Geometry check sheet. Reference: the model listing, model coordinates, mm. Face numbers are marked on the shaded views. A direction names the side the tool comes from. Coordinates: 2 decimals unless noted, no trailing zeros. Write each loop counter-clockwise with the first axis right and the second up, starting at its lowest first coordinate (ties: lowest second). Pieces come first, ordered by that corner, then holes. Notation, with made-up numbers: (0.5, 52) -> (5.5, 52) arc R28 cw to (5.5, 82) -> close; hole circle Ø9 at (-29, -38). An arc over 180 degrees is marked (long way). Answer as CSV lines item,"result".
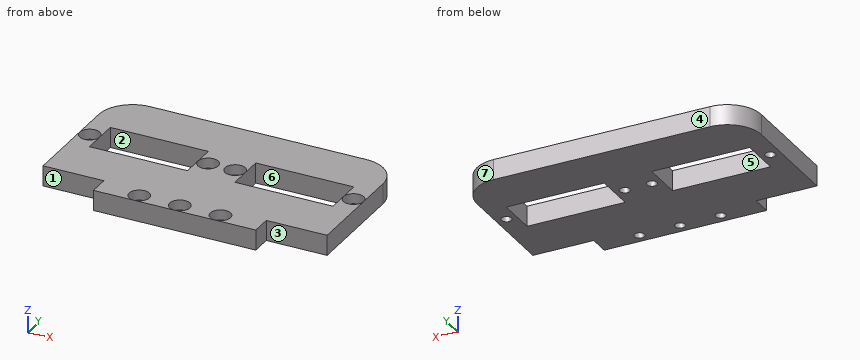
```python
from build123d import *

# Parameters (mm, degrees)
ESQUISSE2_W             = 84
ESQUISSE2_H             = 48
BOSS_EXTRU_1_DEPTH      = 6
ESQUISSE3_R             = 1.5
ESQUISSE3_W             = 18
ESQUISSE3_H             = 6
ESQUISSE3_W_2           = 29
ESQUISSE3_H_2           = 12
ENL_V_MAT_EXTRU_1_DEPTH = 6
ESQUISSE4_R             = 2.995
ENL_V_MAT_EXTRU_2_DEPTH = 3
CONG_1_R                = 10


with BuildPart() as part:
    # Esquisse2 → Boss.-Extru.1 (new body)
    with BuildSketch(Plane.XY):
        with Locations((10.587382635, 10.131926121)):
            Rectangle(ESQUISSE2_W, ESQUISSE2_H)
    extrude(amount=BOSS_EXTRU_1_DEPTH)

    # Esquisse3 → Enlèv. mat.-Extru.1 (cut)
    with BuildSketch(Plane.XY.offset(6)):
        with Locations((-28.412617365, 13.131926121)):
            Circle(ESQUISSE3_R)
        with Locations((49.587382635, 13.131926121)):
            Circle(ESQUISSE3_R)
        with Locations((6.587382635, 13.131926121)):
            Circle(ESQUISSE3_R)
        with Locations((14.587382635, 13.131926121)):
            Circle(ESQUISSE3_R)
        with Locations((-1.412617365, -10.868073879)):
            Circle(ESQUISSE3_R)
        with Locations(Location((22.587382635, -10.868073879, 0), (0, 0, 180))):
            Circle(ESQUISSE3_R)
        with Locations((10.587382635, -10.868073879)):
            Circle(ESQUISSE3_R)
        with Locations((-22.412617365, -10.868073879)):
            Rectangle(ESQUISSE3_W, ESQUISSE3_H)
        with Locations((43.587382635, -10.868073879)):
            Rectangle(ESQUISSE3_W, ESQUISSE3_H)
        with Locations((-10.912617365, 13.131926121)):
            Rectangle(ESQUISSE3_W_2, ESQUISSE3_H_2)
        with Locations((32.087382635, 13.131926121)):
            Rectangle(ESQUISSE3_W_2, ESQUISSE3_H_2)
    extrude(amount=-ENL_V_MAT_EXTRU_1_DEPTH, mode=Mode.SUBTRACT)

    # Esquisse4 → Enlèv. mat.-Extru.2 (cut)
    with BuildSketch(Plane.XY.offset(6)):
        with Locations((-1.412617365, -10.868073879)):
            Circle(ESQUISSE4_R)
        with Locations((22.587382635, -10.868073879)):
            Circle(ESQUISSE4_R)
        with Locations((10.587382635, -10.868073879)):
            Circle(ESQUISSE4_R)
        with Locations((-28.412617365, 13.131926121)):
            Circle(ESQUISSE4_R)
        with Locations((6.587382635, 13.131926121)):
            Circle(ESQUISSE4_R)
        with Locations((14.587382635, 13.131926121)):
            Circle(ESQUISSE4_R)
        with Locations((49.587382635, 13.131926121)):
            Circle(ESQUISSE4_R)
    extrude(amount=-ENL_V_MAT_EXTRU_2_DEPTH, mode=Mode.SUBTRACT)

    # Congé1
    cong_1_edges = [part.edges().sort_by_distance(p)[0] for p in [
        (-31.412617365, 34.131926121, 3),
        (52.587382635, 34.131926121, 3),
    ]]
    fillet(cong_1_edges, radius=CONG_1_R)


solid = part.part
```
Item 1: Cross-section at C-C, the plane y = 31. Record the cut outline in (x, z), plus the area to 3 significant figures.
Responses:
outline,"(-28.68, 0) -> (49.86, 0) -> (49.86, 6) -> (-28.68, 6) -> close"
area,"471 mm2"
Item 2: Depth check by flat-ended pin: pin 1 Ø5 at (x, y) = (-1, -11) entering from +Z; pin 2 Ø1.5 at (x, z) = (-23, 1) entering from +Y. Enter the tip coordinate at first touch or a pass-through.
Responses:
pin 1,"stops at z = 3"
pin 2,"stops at y = 34.1"
Item 3: Thickness scan on probe 1 along Y at (x, z) = (3.5, 4.35); probe 2 along Y at (x, z) = (-18.5, 2.4); probe 3 along X at (y, z) = (10, 0.85). Record the ranges inside material, lowest first.
Responses:
probe 1,"y = -13.87 to 7.13, 19.13 to 34.13"
probe 2,"y = -7.87 to 7.13, 19.13 to 34.13"
probe 3,"x = -31.41 to -25.41, 3.59 to 17.59, 46.59 to 52.59"
Item 4: Set-up check for the marked faces 1, 2 and 3: record each of +Z, -Z, +X, -X, +Y, -Y from which the full face is reachable in a straight line by a thin tool's end or side.
Responses:
face 1,"+Z, -Z, -X, -Y"
face 2,"+Z, -Z"
face 3,"+Z, -Z, +X, -Y"
Item 5: Cross-section at B-B, the plane z = 2.2. Count the separate pieces of the cut face and the enclosed holes in it, plus the area to 3 significant figures.
Responses:
separate pieces,"1"
enclosed holes,"9"
area,"3,030 mm2"
Item 6: Release check for a two-part mould opening along X. For the marked faces 4, 5, 6 and 7 record: +X half, -X half, draft (parallel to the pull), parting line (faces both ways), or undercut.
Responses:
face 4,"draft"
face 5,"undercut"
face 6,"undercut"
face 7,"+X half"
Item 7: Cross-section at A-A, the plane x = -6.5. Record the cut outline in (y, z).
Responses:
outline,"(-13.87, 0) -> (7.13, 0) -> (7.13, 6) -> (-13.87, 6) -> close; (19.13, 0) -> (34.13, 0) -> (34.13, 6) -> (19.13, 6) -> close"
